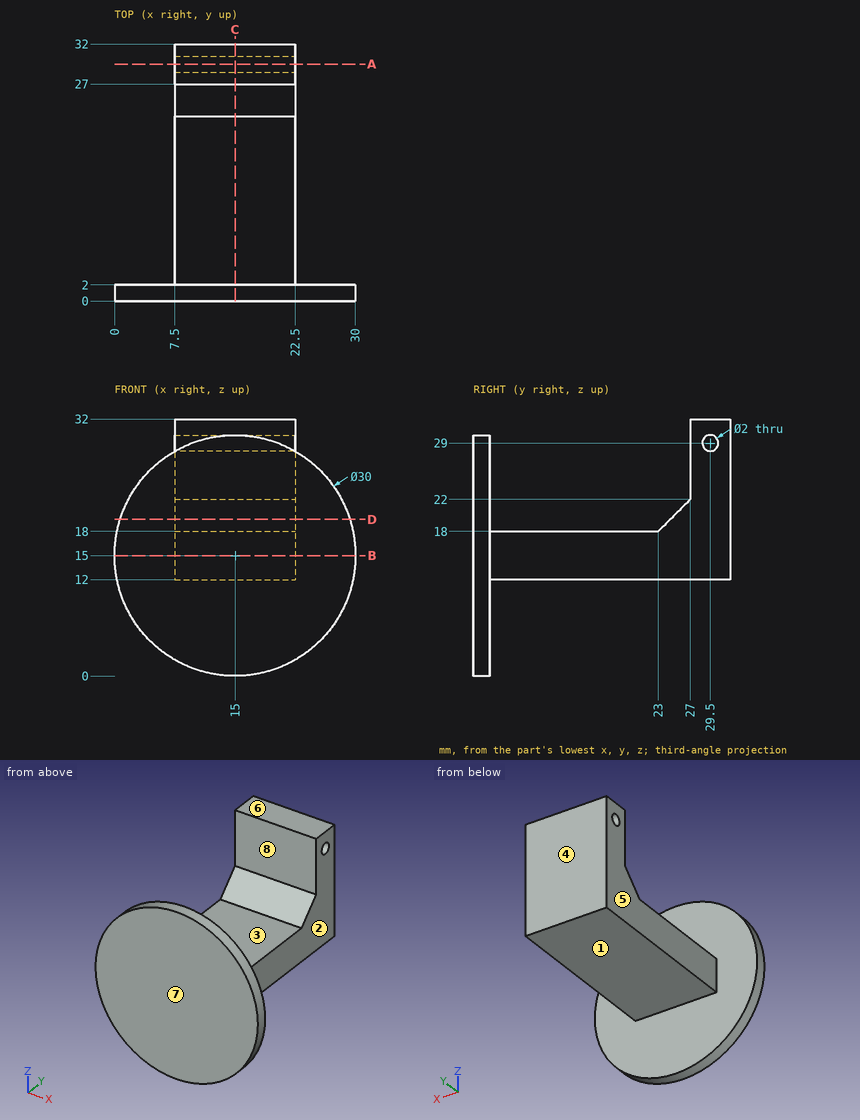
Drawing for the job (mm, zero at the part's lowest x, y, z). A direction names the side the tool comes from. Round coordinates to 2 decimals unless told otherwise and drop trailing zeros. Write each loop counter-clockwise with the first axis right and the second up, starting at its lowest first coordinate (ties: lowest second). Pieces come first, ordered by that corner, then holes. Notation, with made-up numbers: M -38,18.5 L -29,18.5 A24 cw -29,28.5 Z; hole C 51.25,-3 d9. An arc over 180 degrees is marked long. Put each result on its own line as item: value.
Item 1: Cut at B-B (z = 15). List the corners of the cut face in (x, y).
Responses:
outline: M 0,0 L 30,0 L 30,2 L 22.5,2 L 22.5,32 L 7.5,32 L 7.5,2 L 0,2 Z
Item 2: Flat gauge pins, fed straight in: P1, Ø10, axis at x = 8.5, y = 10, coming from the -Z side; P2, Ø3, axis at y = 29.5, z = 29, coming from the -X side; P3, Ø4.5, axis at x = 15.5, y = 13.5, coming from the +Z side. Where does each tip first touch, or does it go through?
Responses:
P1: z = 12
P2: x = 7.5
P3: z = 18
Item 3: Tool access for the marked faces 1, 2, 3, 4 and 5: list every direction of +Z, -Z, +X, -X, +Y, -Y with a clear straight run to the whole face (end or side of a thin tool).
Responses:
face 1: -Z, +X, -X, +Y
face 2: +Z, -Z, +X, +Y
face 3: +Z, +X, -X
face 4: +Z, -Z, +X, -X, +Y
face 5: +Z, -Z, -X, +Y
Item 4: Mould opens along Y. For the marked faces 6, 7 and 8 say: +Y half, -Y half, draft (parallel to the pull), parting line (faces both ways), or undercut.
Responses:
face 6: draft
face 7: -Y half
face 8: undercut
Item 5: Cut at A-A (y = 29.5). List the corners of the cut face in (x, z).
Responses:
outline: M 7.5,12 L 22.5,12 L 22.5,28 L 7.5,28 Z; M 7.5,30 L 22.5,30 L 22.5,32 L 7.5,32 Z
Item 6: Cut at C-C (x = 15). List the corners of the cut face in (y, z).
Responses:
outline: M 0,0 L 2,0 L 2,12 L 32,12 L 32,32 L 27,32 L 27,22 L 23,18 L 2,18 L 2,30 L 0,30 Z; hole C 29.5,29 d2
Item 7: Probe L1, parallel to Y at x = 13.25, z = 29; L2, parallel to X at y = 28, z = 16; L3, parallel to Z at x = 13.75, y = 12. List the from-to ranges inside material, lowest first. Write a range as from..to.
Responses:
L1: 0..2, 27..28.5, 30.5..32
L2: 7.5..22.5
L3: 12..18
Item 8: Cut at D-D (z = 19.5). List the corners of the cut face in (x, y), and give its area (3 significant figures).
Responses:
outline: M 0.69,0 L 29.31,0 L 29.31,2 L 0.69,2 Z; M 7.5,24.5 L 22.5,24.5 L 22.5,32 L 7.5,32 Z
area: 170 mm²
